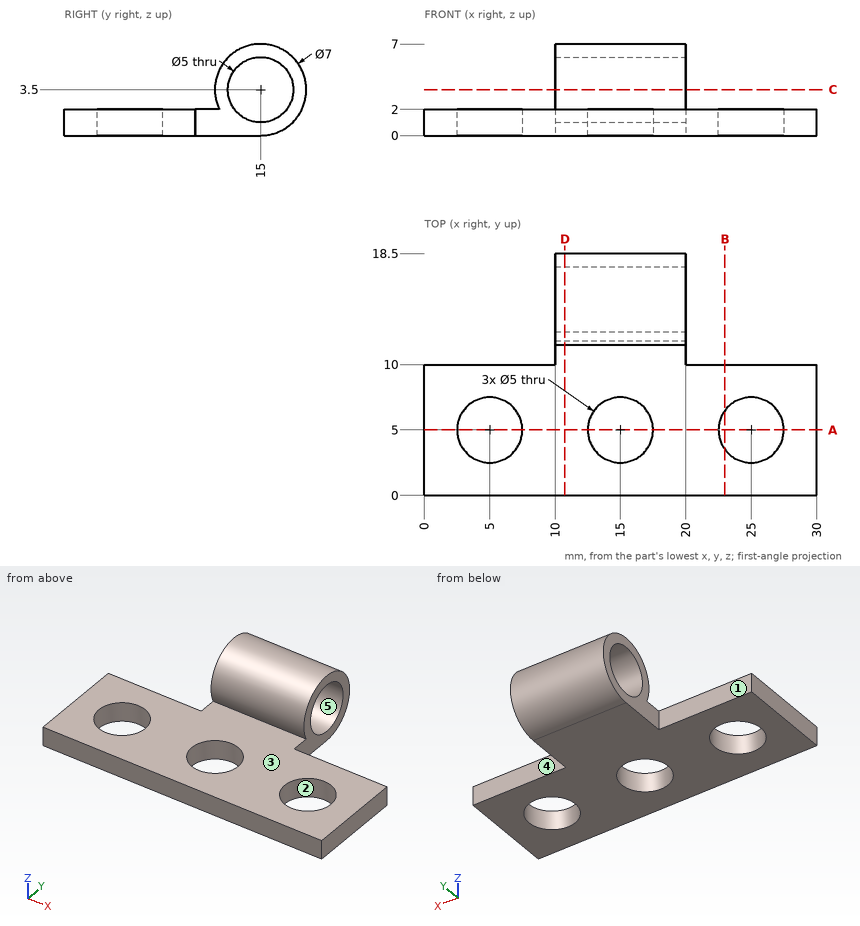
Geometry check sheet. Reference: drawing and pictorial views, mm from the part's lowest x, y, z. A direction names the side the tool comes from. Round coordinates to 2 decimals unless told otherwise and drop trailing zeros. Order: outer loops, then holes, each group sorted by start corner. A loop starts at its lowest first (then second) coordinate and runs counter-clockwise, first axis right, second up. Notation, with made-up numbers: (-9, 66) -> (42, 66) arc R25 ccw to (42, 83) -> close; hole circle Ø5 at (-10, -38.5). An arc over 180 degrees is marked (long way). One line per item, written item: value. Start each with the question number.
Q1. Set-up check for the marked faces 4 and 5: record each of +Z, -Z, +X, -X, +Y, -Y from which the full face is reachable in a straight line by a thin tool's end or side.
Q2. Cross-section at D-D (x = 10.75). Record the boundary of the cut face in (y, z), and give its area (3 significant figures).
Q3. Cross-section at C-C (z = 3.5). Record the boundary of the cut face in (x, y).
Q4. Gauge pin test, flat ends, axial feed: pin 1 Ø6 at (x, y) = (16, 5) entering from +Z; pin 2 Ø0.6 at (x, z) = (6, 1) entering from +Y; pin 3 Ø4 at (y, z) = (15, 3.5) entering from +X; pin 4 Ø8 at (x, y) = (18.5, 9.5) entering from +Z. Record the tip position at first contact, or that the pin passes through.
Q5. Cross-section at B-B (x = 23). Record the boundary of the cut face in (y, z).
Q6. Cross-section at A-A (y = 5). Record the boundary of the cut face in (x, z), and give its area (3 significant figures).
Q7. Thickness scan on line 1 (Y direction, x = 25, z = 0.6); line 2 (X direction, y = 11, z = 0.5); line 3 (Y direction, x = 15, z = 1.6). Record the ranges inside material, lowest first.
Q8. Mould release check, pull along Y, two halves, no side actions. Record for the marked faces 1, 2 and 3: pulls with the +Y half, pulls with the -Y half, needs draft (parallel to the pull), parting line crosses it, or undercut.
Completed:
1. face 4: +Z, -Z, +X, +Y
1. face 5: +X, -X
2. outline: (0, 0) -> (15, 0) arc R3.5 ccw (long way) to (11.84, 2) -> (0, 2) -> close; hole circle Ø5 at (15, 3.5)
2. area: 44.3 mm²
3. outline: (10, 11.5) -> (20, 11.5) -> (20, 12.5) -> (10, 12.5) -> close; (10, 17.5) -> (20, 17.5) -> (20, 18.5) -> (10, 18.5) -> close
4. pin 1: stops at z = 2
4. pin 2: stops at y = 10
4. pin 3: passes through
4. pin 4: stops at z = 6.66
5. outline: (0, 0) -> (3.5, 0) -> (3.5, 2) -> (0, 2) -> close; (6.5, 0) -> (10, 0) -> (10, 2) -> (6.5, 2) -> close
6. outline: (0, 0) -> (2.5, 0) -> (2.5, 2) -> (0, 2) -> close; (7.5, 0) -> (12.5, 0) -> (12.5, 2) -> (7.5, 2) -> close; (17.5, 0) -> (22.5, 0) -> (22.5, 2) -> (17.5, 2) -> close; (27.5, 0) -> (30, 0) -> (30, 2) -> (27.5, 2) -> close
6. area: 30.0 mm²
7. line 1: y = 0 to 2.5, 7.5 to 10
7. line 2: x = 10 to 20
7. line 3: y = 0 to 2.5, 7.5 to 13.38, 16.62 to 17.94
8. face 1: pulls with the +Y half
8. face 2: undercut
8. face 3: needs draft
